```python
from build123d import *

# Parameters (mm, degrees)
BOSS_EXTRUDE1_DEPTH = 8
MOVE_FACE1_BY       = 19
SKETCH3_R           = 1.55
CUT_EXTRUDE1_DEPTH  = 99.460415825


with BuildPart() as part:
    # Sketch2 → Boss-Extrude1 (new, symmetric)
    with BuildSketch(Plane.XZ):
        Polygon((-13.796187154, 46.508213699), (-13.796187154, -23.491786301), (-48.796187154, -23.491786301), (-48.796187154, 11.508213699), (-104.296187154, 11.508213699), (-104.296187154, 46.508213699), align=None)
    extrude(amount=BOSS_EXTRUDE1_DEPTH, both=True)

    # Move Face1: a face moved inward by 19.0
    extrude(part.faces().sort_by_distance((-104.296187154, 0, 29.008213699))[0], amount=MOVE_FACE1_BY, dir=(1, 0, 0), mode=Mode.SUBTRACT)

    # Sketch3 → Cut-Extrude1 (cut, through all)
    with BuildSketch(Plane.XZ.offset(8)):
        with Locations(Location((-16.646187154, 44.158213699, 0), (0, 0, 270))):
            Circle(SKETCH3_R)
        with Locations(Location((-16.646187154, -21.541786301, 0), (0, 0, 270))):
            Circle(SKETCH3_R)
    extrude(amount=-CUT_EXTRUDE1_DEPTH, mode=Mode.SUBTRACT)


solid = part.part
```
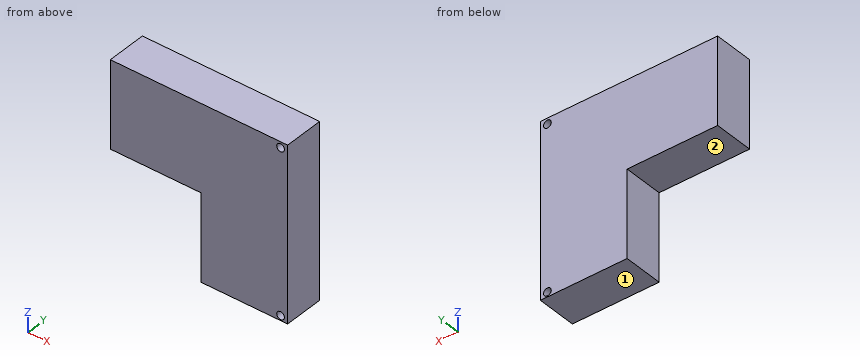
The model under review builds one solid part; all positions refer to its coordinate system, in mm. Face numbers are marked on the shaded views. A direction names the side the tool comes from. Round coordinates to 2 decimals unless told otherwise and drop trailing zeros. Loops run counter-clockwise (first coordinate to the right, second up) from the corner with the lowest first, then second, coordinate; pieces in that order, holes last. Notation, with made-up numbers: (9.25, 87.25) - (63.25, 87.25) arc R13 ccw to (63.25, 91.25) - close; hole circle Ø1 at (14.5, 71.25). An arc over 180 degrees is marked (long way). Write each question's results on one line, items separated by ' | '. Start each with the question number.
Q1. Take a section at A-A on y = -2.75. Give the boundary of the cut face in (x, z), plus the area to 3 significant figures.
Q2. Insertion check: P1, Ø8, axis at x = -59, y = -3, coming from the -Z side; P2, Ø3, axis at x = -16.65, z = -21.54, coming from the +Y side. Each pin has a flat end and moves straight along its axis. Give the tip position at first contact, or say it passes through.
Q3. Take a section at C-C on z = -16. Give the boundary of the cut face in (x, y), plus the area to 3 significant figures.
Q4. Take a section at B-B on x = -51.5. Give the boundary of the cut face in (y, z), plus the area to 3 significant figures.
Q5. Wall thickness on line 1 along Z through (x, y) = (-53, 2.25); line 2 along X through (y, z) = (0.25, -0.5): over which ranges is each line inside the solid? List them lowest first. Write a range as [from, to].
Q6. Tool access review of the marked faces 1 and 2: name each direction out of +Z, -Z, +X, -X, +Y, -Y from which nothing blocks a thin tool from reaching the whole face with its end or side.
Data:
1) outline: (-85.3, 11.51) - (-48.8, 11.51) - (-48.8, -23.49) - (-13.8, -23.49) - (-13.8, 46.51) - (-85.3, 46.51) - close; hole circle Ø3.1 at (-16.65, -21.54); hole circle Ø3.1 at (-16.65, 44.16) | area: 3,710 mm²
2) P1: stops at z = 11.51 | P2: passes through
3) outline: (-48.8, -8) - (-13.8, -8) - (-13.8, 8) - (-48.8, 8) - close | area: 560 mm²
4) outline: (-8, 11.51) - (8, 11.51) - (8, 46.51) - (-8, 46.51) - close | area: 560 mm²
5) line 1: z = [11.51, 46.51] | line 2: x = [-48.8, -13.8]
6) face 1: -Z, +X, -X, +Y, -Y | face 2: -Z, -X, +Y, -Y
